Can you work these out from the model? Positions are in its coordinate system, mm. Face numbers are marked on the shaded views. A direction names the side the tool comes from. Give positions to 0.01 mm unless a question says otherwise; leave off trailing zeros. Write each loop counter-clockwise with the first axis right and the second up, starting at its lowest first coordinate (ties: lowest second). Pieces come first, ordered by that corner, then holes. Notation, with made-up numbers: (-7, 60) -> (28, 60) arc R8 cw to (28, 64) -> close; hole circle Ø7 at (85.5, -11.75). An arc over 180 degrees is marked (long way). One line per item, written item: value.
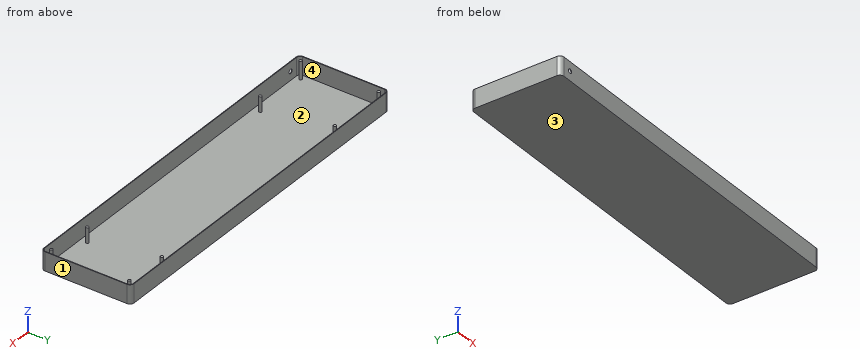
from build123d import *

# Parameters (mm, degrees)
BOSS_EXTRU_1_DEPTH      = 50.5
BOSS_EXTRU_2_DEPTH      = 2
ESQUISSE6_R             = 4
BOSS_EXTRU_4_DEPTH      = 50.5
ESQUISSE7_R             = 4
BOSS_EXTRU_5_DEPTH      = 42.5
ESQUISSE8_R             = 6
ENL_V_MAT_EXTRU_1_DEPTH = 2


with BuildPart() as part:
    # Esquisse2 → Boss.-Extru.1 (new body)
    with BuildSketch(Plane.XY):
        with BuildLine():
            Line((694.77885805, 135.537159381), (-285.22114195, 135.537159381))
            ThreePointArc((-285.22114195, 135.537159381), (-293.706423325, 132.022440755), (-297.22114195, 123.537159381))
            Line((-297.22114195, 123.537159381), (-297.22114195, -106.462840619))
            ThreePointArc((-297.22114195, -106.462840619), (-293.706423325, -114.948121993), (-285.22114195, -118.462840619))
            Line((-285.22114195, -118.462840619), (694.77885805, -118.462840619))
            ThreePointArc((694.77885805, -118.462840619), (703.264139424, -114.948121993), (706.77885805, -106.462840619))
            Line((706.77885805, -106.462840619), (706.77885805, 123.537159381))
            ThreePointArc((706.77885805, 123.537159381), (703.264139424, 132.022440755), (694.77885805, 135.537159381))
        make_face()
        with BuildLine():
            Line((-295.22114195, 123.537159381), (-295.22114195, -106.462840619))
            ThreePointArc((-295.22114195, -106.462840619), (-292.292209762, -113.533908431), (-285.22114195, -116.462840619))
            Line((-285.22114195, -116.462840619), (694.77885805, -116.462840619))
            ThreePointArc((694.77885805, -116.462840619), (701.849925862, -113.533908431), (704.77885805, -106.462840619))
            Line((704.77885805, -106.462840619), (704.77885805, 123.537159381))
            ThreePointArc((704.77885805, 123.537159381), (701.849925862, 130.608227193), (694.77885805, 133.537159381))
            Line((694.77885805, 133.537159381), (-285.22114195, 133.537159381))
            ThreePointArc((-285.22114195, 133.537159381), (-292.292209762, 130.608227193), (-295.22114195, 123.537159381))
        make_face(mode=Mode.SUBTRACT)
    extrude(amount=-BOSS_EXTRU_1_DEPTH)

    # Esquisse4 → Boss.-Extru.2 (add)
    with BuildSketch(Plane(origin=(0, 0, -50.5), x_dir=(-1, 0, 0), z_dir=(0, 0, -1))):
        with BuildLine():
            Line((297.22114195, 123.537159381), (297.22114195, -106.462840619))
            ThreePointArc((297.22114195, -106.462840619), (293.706423325, -114.948121993), (285.22114195, -118.462840619))
            Line((285.22114195, -118.462840619), (-694.77885805, -118.462840619))
            ThreePointArc((-694.77885805, -118.462840619), (-703.264139424, -114.948121993), (-706.77885805, -106.462840619))
            Line((-706.77885805, -106.462840619), (-706.77885805, 123.537159381))
            ThreePointArc((-706.77885805, 123.537159381), (-703.264139424, 132.022440755), (-694.77885805, 135.537159381))
            Line((-694.77885805, 135.537159381), (285.22114195, 135.537159381))
            ThreePointArc((285.22114195, 135.537159381), (293.706423325, 132.022440755), (297.22114195, 123.537159381))
        make_face()
    extrude(amount=BOSS_EXTRU_2_DEPTH)

    # Esquisse6 → Boss.-Extru.4 (add)
    with BuildSketch(Plane.XY.offset(-50.5)):
        with Locations(Location((-280.22114195, 118.537159381, 0), (0, 0, 180))):
            Circle(ESQUISSE6_R)
        with Locations(Location((-280.22114195, -101.462840619, 0), (0, 0, 180))):
            Circle(ESQUISSE6_R)
        with Locations(Location((689.77885805, -101.462840619, 0), (0, 0, 180))):
            Circle(ESQUISSE6_R)
        with Locations(Location((689.77885805, 118.537159381, 0), (0, 0, 180))):
            Circle(ESQUISSE6_R)
    extrude(amount=BOSS_EXTRU_4_DEPTH)

    # Esquisse7 → Boss.-Extru.5 (add)
    with BuildSketch(Plane.XY.offset(-50.5)):
        with Locations(Location((-116.842462294, 113.537159381, 0), (0, 0, 180))):
            Circle(ESQUISSE7_R)
        with Locations(Location((-116.842462294, -96.462840619, 0), (0, 0, 180))):
            Circle(ESQUISSE7_R)
        with Locations(Location((556.289518221, 113.537159381, 0), (0, 0, 180))):
            Circle(ESQUISSE7_R)
        with Locations(Location((556.289518221, -96.462840619, 0), (0, 0, 180))):
            Circle(ESQUISSE7_R)
    extrude(amount=BOSS_EXTRU_5_DEPTH)

    # Esquisse8 → Enlèv. mat.-Extru.1 (cut)
    with BuildSketch(Plane(origin=(0, -118.462840619, 0), x_dir=(-1, 0, 0), z_dir=(0, -1, 0))):
        with Locations(Location((262.22114195, 26.25, 0), (0, 0, 90))):
            Circle(ESQUISSE8_R)
    extrude(amount=-ENL_V_MAT_EXTRU_1_DEPTH, mode=Mode.SUBTRACT)


solid = part.part
1) Will these pins go through, and if not, where does the flat tip stop? pin 1 (6 mm diameter, centred on x = 434, y = -35.5, fed in from +Z); pin 2 (7 mm diameter, centred on x = -262.22, z = -26.25, fed in from -Y); pin 3 (2.5 mm diameter, centred on x = 557.5, y = 113.5, fed in from +Z).
Answer list:
pin 1: stops at z = -50.5
pin 2: stops at y = 133.54
pin 3: stops at z = -8
2) I need wall thicknesses on L1, parallel to X at y = 93, z = -28; L2, parallel to Y at x = 328, z = -44; L3, parallel to Z at x = -99, y = -74. Which ranges of each line are inside material? Lowest first, please.
Answer list:
L1: x = -297.22 to -295.22, 704.78 to 706.78
L2: y = -118.46 to -116.46, 133.54 to 135.54
L3: z = -52.5 to -50.5
3) For the marked faces 3 and 4, which set-ups out of +Z, -Z, +X, -X, +Y, -Y let a thin tool reach every point of the face, with its end or its side?
Answer list:
face 3: -Z, +X, -X, +Y, -Y
face 4: +Z
4) If we section it at C-C (y = 78.5): Write out the boundary of the cut face in (x, z).
Answer list:
outline: (-297.22, -52.5) -> (706.78, -52.5) -> (706.78, 0) -> (704.78, 0) -> (704.78, -50.5) -> (-295.22, -50.5) -> (-295.22, 0) -> (-297.22, 0) -> close
5) We'd pull the mould along Y, two halves only. Please class the marked faces 1 and 2: released by +Y, released by -Y, zero draft, split by the parting line, or undercut.
Answer list:
face 1: zero draft
face 2: undercut
6) If we section it at B-B (x = 187.5): Write out the boundary of the cut face in (y, z).
Answer list:
outline: (-118.46, -52.5) -> (135.54, -52.5) -> (135.54, 0) -> (133.54, 0) -> (133.54, -50.5) -> (-116.46, -50.5) -> (-116.46, 0) -> (-118.46, 0) -> close
7) If we section it at A-A (z = -41.5): State how many separate pieces and enclosed holes the cut face has, and give its area (3 significant figures).
Answer list:
separate pieces: 9
enclosed holes: 1
area: 5,380 mm^2
